For this review, take the finished solid that the model builds, in its own axes (mm). Round coordinates to 2 decimals unless told otherwise and drop trailing zeros. Order: outer loops, then holes, each group sorted by start corner. A loop starts at its lowest first (then second) coordinate and runs counter-clockwise, first axis right, second up. Notation, with made-up numbers: (11.5, -23) - (37.5, -23) arc R6 cw to (37.5, -15) - close; hole circle Ø11 at (-15, 23.5). An arc over 180 degrees is marked (long way). One line per question, with ' | ' between items.
```python
from build123d import *

# Parameters (mm, degrees)
F0_W     = 100
F0_H     = 24
F1_DEPTH = 22
F2_R     = 4
F3_DEPTH = 24.001
F4_SIZE  = 0.5
F5_W     = 100
F5_H     = 24
F6_DEPTH = 35
F7_R     = 3
F8_DEPTH = 24.001
F9_SIZE  = 0.5


with BuildPart() as f1:
    # F0 (on Right) → F1 (new body)
    with BuildSketch(Plane.YZ):
        Rectangle(F0_W, F0_H)
    extrude(amount=-F1_DEPTH)

    # F2 (on face) → F3 (cut, through all)
    with BuildSketch(Plane.XY.offset(12)):
        with Locations((-8, 28)):
            Circle(F2_R)
        with Locations((-8, -32)):
            Circle(F2_R)
    extrude(amount=-F3_DEPTH, mode=Mode.SUBTRACT)

    # F4
    f4_edges = [f1.edges().sort_by_distance(p)[0] for p in [
        (-12, 28, 12),
        (-4, 28, 0),
        (-12, 28, -12),
        (-12, -32, 12),
        (-4, -32, 0),
        (-12, -32, -12),
    ]]
    chamfer(f4_edges, length=F4_SIZE)

    # F5 (on face) → F6 (join)
    with BuildSketch(Plane.YZ):
        Rectangle(F5_W, F5_H)
    extrude(amount=F6_DEPTH)

    # F7 (on face) → F8 (cut, through all)
    with BuildSketch(Plane.XY.offset(12)):
        with Locations((27, 5)):
            Circle(F7_R)
        with Locations((27, 35)):
            Circle(F7_R)
        with Locations((12, 35)):
            Circle(F7_R)
        with Locations((12, 5)):
            Circle(F7_R)
    extrude(amount=-F8_DEPTH, mode=Mode.SUBTRACT)

    # F9
    f9_edges = [f1.edges().sort_by_distance(p)[0] for p in [
        (24, 5, 12),
        (30, 5, 0),
        (24, 5, -12),
        (24, 35, 12),
        (30, 35, 0),
        (24, 35, -12),
        (9, 35, 12),
        (15, 35, 0),
        (9, 35, -12),
        (9, 5, 12),
        (15, 5, 0),
        (9, 5, -12),
    ]]
    chamfer(f9_edges, length=F9_SIZE)


solid = f1.part
```
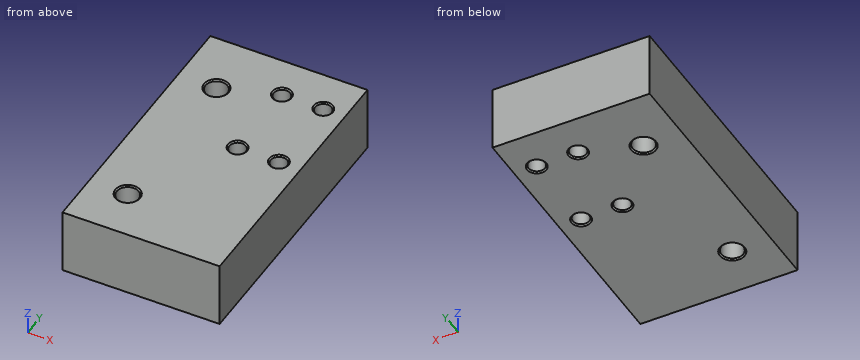
(1) For probe 1 along Y at (x, z) = (27, 6.25); probe 2 along Y at (x, z) = (-8, 0), list the stretches that pass through material, from the lowest coordinate up. Write a range as [from, to].
Output values:
probe 1: [-50, 2], [8, 32], [38, 50] | probe 2: [-50, -36], [-28, 24], [32, 50]
(2) We need section B-B on x = 27. State the section outline as (y, z) points, plus the area to 3 significant figures.
Output values:
outline: (-50, -12) - (1.5, -12) - (2, -11.5) - (2, 11.5) - (1.5, 12) - (-50, 12) - close; (8, -11.5) - (8.5, -12) - (31.5, -12) - (32, -11.5) - (32, 11.5) - (31.5, 12) - (8.5, 12) - (8, 11.5) - close; (38, -11.5) - (38.5, -12) - (50, -12) - (50, 12) - (38.5, 12) - (38, 11.5) - close | area: 2,110 mm^2
(3) We need section C-C on z = 4.75. State the section outline as (x, y) points, plus the area to 3 significant figures.
Output values:
outline: (-22, -50) - (35, -50) - (35, 50) - (-22, 50) - close; hole circle Ø8 at (-8, -32); hole circle Ø8 at (-8, 28); hole circle Ø6 at (12, 5); hole circle Ø6 at (12, 35); hole circle Ø6 at (27, 5); hole circle Ø6 at (27, 35) | area: 5,490 mm^2
(4) Insertion check: pin 1 (7 mm diameter, centred on x = -8, y = 28, fed in from -Z); pin 2 (9.5 mm diameter, centred on x = 27, y = 5, fed in from +Z); pin 3 (1 mm diameter, centred on x = -11.5, y = -30.5, fed in from -Z). Each pin has a flat end and moves straight along its axis. Give the tip position at first contact, or say it passes through.
Output values:
pin 1: through | pin 2: z = 12 | pin 3: z = -11.81
(5) We need section A-A on y = 35. State the section outline as (x, z) points, plus the area to 3 significant figures.
Output values:
outline: (-22, -12) - (8.5, -12) - (9, -11.5) - (9, 11.5) - (8.5, 12) - (-22, 12) - close; (15, -11.5) - (15.5, -12) - (23.5, -12) - (24, -11.5) - (24, 11.5) - (23.5, 12) - (15.5, 12) - (15, 11.5) - close; (30, -11.5) - (30.5, -12) - (35, -12) - (35, 12) - (30.5, 12) - (30, 11.5) - close | area: 1,080 mm^2
